```python
from build123d import *

# Parameters (mm, degrees)
ESBO_O1_W                  = 25
ESBO_O1_H                  = 65
ESBO_O1_R                  = 1.75
RESSALTO_EXTRUS_O1_DEPTH   = 5
CORTE_EXTRUS_O3_DEPTH      = 36.178118199
CORTE_EXTRUS_O3_DEPTH_BACK = 36.178118199
FILETE1_R                  = 5
ESBO_O2_R                  = 3.4
CORTE_EXTRUS_O1_DEPTH      = 3
ESBO_O3_W                  = 5.6
ESBO_O3_H                  = 48
CORTE_EXTRUS_O2_DEPTH      = 3


with BuildPart() as part:
    # Esboço1 → Ressalto-extrusão1 (new body)
    with BuildSketch(Plane.XY):
        Rectangle(ESBO_O1_W, ESBO_O1_H)
        with Locations((7.5, 27.5)):
            Circle(ESBO_O1_R, mode=Mode.SUBTRACT)
        with Locations(Location((7.5, -27.5, 0), (0, 0, 180))):
            Circle(ESBO_O1_R, mode=Mode.SUBTRACT)
        with Locations((-7.5, -27.5)):
            Circle(ESBO_O1_R, mode=Mode.SUBTRACT)
        with Locations(Location((-7.5, 27.5, 0), (0, 0, 180))):
            Circle(ESBO_O1_R, mode=Mode.SUBTRACT)
        with BuildLine():
            Line((-1.7, -20), (-1.7, 20))
            ThreePointArc((-1.7, 20), (0, 21.7), (1.7, 20))
            Line((1.7, 20), (1.7, -20))
            ThreePointArc((1.7, -20), (0, -21.7), (-1.7, -20))
        make_face(mode=Mode.SUBTRACT)
    extrude(amount=RESSALTO_EXTRUS_O1_DEPTH)

    # Esboço4 → Corte-extrusão3 (cut, two sides: drawn at the far end of the back side and taken through both)
    with BuildSketch(Plane.XY.offset(5).offset(-CORTE_EXTRUS_O3_DEPTH_BACK)):
        with BuildLine():
            Line((12.5, 27.5), (12.5, -27.5))
            ThreePointArc((12.5, -27.5), (12.365923064, -26.34987273), (11.970882905, -25.261427677))
            ThreePointArc((11.970882905, -25.261427677), (6, 0), (11.970882905, 25.261427677))
            ThreePointArc((11.970882905, 25.261427677), (12.365923064, 26.34987273), (12.5, 27.5))
        make_face()
        with BuildLine():
            Line((-12.5, 27.5), (-12.5, -27.5))
            ThreePointArc((-12.5, -27.5), (-12.365923064, -26.34987273), (-11.970882905, -25.261427677))
            ThreePointArc((-11.970882905, -25.261427677), (-6, 0), (-11.970882905, 25.261427677))
            ThreePointArc((-11.970882905, 25.261427677), (-12.365923064, 26.34987273), (-12.5, 27.5))
        make_face()
    extrude(amount=CORTE_EXTRUS_O3_DEPTH + CORTE_EXTRUS_O3_DEPTH_BACK, mode=Mode.SUBTRACT)

    # Filete1
    filete1_edges = [part.edges().sort_by_distance(p)[0] for p in [
        (-12.5, -32.5, 2.5),
        (12.5, -32.5, 2.5),
        (12.5, 32.5, 2.5),
        (-12.5, 32.5, 2.5),
    ]]
    fillet(filete1_edges, radius=FILETE1_R - 0.0001)  # a hair under: the kernel refuses the full size

    # Esboço2 → Corte-extrusão1 (cut)
    with BuildSketch(Plane.XY.offset(5)):
        with Locations((7.5, 27.5)):
            Circle(ESBO_O2_R)
        with Locations((-7.5, 27.5)):
            Circle(ESBO_O2_R)
        with Locations((-7.5, -27.5)):
            Circle(ESBO_O2_R)
        with Locations((7.5, -27.5)):
            Circle(ESBO_O2_R)
    extrude(amount=-CORTE_EXTRUS_O1_DEPTH, mode=Mode.SUBTRACT)

    # Esboço3 → Corte-extrusão2 (cut)
    with BuildSketch(Plane(origin=(0, 0, 0), x_dir=(-1, 0, 0), z_dir=(0, 0, -1))):
        Rectangle(ESBO_O3_W, ESBO_O3_H)
    extrude(amount=-CORTE_EXTRUS_O2_DEPTH, mode=Mode.SUBTRACT)


solid = part.part
```
The model under review builds one solid part; all positions refer to its coordinate system, in mm. A direction names the side the tool comes from. Give positions to 0.01 mm unless a question says otherwise; leave off trailing zeros. Write each loop counter-clockwise with the first axis right and the second up, starting at its lowest first coordinate (ties: lowest second). Pieces come first, ordered by that corner, then holes. Notation, with made-up numbers: M 79.25,37 L 103.25,37 A20 ccw 103.25,54 Z; hole C 74.5,50.25 d2. An arc over 180 degrees is marked long. Answer in a Markdown table with one row per item.
Item 1: Add section A-A on z = 4.1. State how many separate pieces and enclosed holes the cut face has, plus the area to 3 significant figures.
Check sheet entries:
| item | result |
|---|---|
| separate pieces | 1 |
| enclosed holes | 5 |
| area | 852 mm2 |
Item 2: For P1, Ø2, axis at y = -14, z = 1, coming from the +X side; P2, Ø2, axis at y = 22, z = 1, coming from the -X side; P3, Ø6, axis at x = -7.5, y = -27.5, coming from the +Z side; P4, Ø3, axis at x = 7.5, y = -27.5, coming from the +Z side, all flat-tipped, find the tip position at first contact; note any pin that passes through.
Check sheet entries:
| item | result |
|---|---|
| P1 | x = 8.03 |
| P2 | x = -10.9 |
| P3 | z = 2 |
| P4 | through |
Item 3: Add section B-B on x = -10. Give the boundary of the cut face in (y, z).
Check sheet entries:
| item | result |
|---|---|
| outline | M -31.83,0 L -20.87,0 L -20.87,5 L -25.2,5 L -25.2,2 L -29.8,2 L -29.8,5 L -31.83,5 Z; M 20.87,0 L 31.83,0 L 31.83,5 L 29.8,5 L 29.8,2 L 25.2,2 L 25.2,5 L 20.87,5 Z |
Item 4: Draft analysis for pull direction Y (two halves, no side actions). For faces 1 (the face through (0, 32.5, 2)), 2 (the face through (12.36, 26.33, 2.47)), 3 (the face through (-11.07, -31, 2.54)), state which applies: +Y half, -Y half, draft (parallel to the pull), parting line (faces both ways), or undercut.
Check sheet entries:
| item | result |
|---|---|
| face 1 | +Y half |
| face 2 | undercut |
| face 3 | -Y half |
Item 5: Tool access review of faces 4 (the face through (12.37, -26.37, 2.47)), 5 (the face through (-12.36, 26.33, 2.47)), 6 (the face through (-1.7, 0, 4)), 7 (the face through (11, -31.07, 2.54)), 8 (the face through (10.743, -26.479, 3.521)): name each direction out of +Z, -Z, +X, -X, +Y, -Y from which nothing blocks a thin tool from reaching the whole face with its end or side.
Check sheet entries:
| item | result |
|---|---|
| face 4 | +Z, -Z, +X |
| face 5 | +Z, -Z, -X |
| face 6 | +Z, -Z |
| face 7 | +Z, -Z, +X, -Y |
| face 8 | +Z |
Item 6: For line 1 along X through (y, z) = (27.5, 1.65); line 2 along Y through (x, z) = (5.5, 4.1); line 3 along Y through (x, z) = (0.5, 0.85), list the stretches that pass through material, from the lowest coordinate up.
Check sheet entries:
| item | result |
|---|---|
| line 1 | -12.5 to -9.25, -5.75 to 5.75, 9.25 to 12.5 |
| line 2 | -32.5 to -30.25, -24.75 to 24.75, 30.25 to 32.5 |
| line 3 | -32.5 to -24, 24 to 32.5 |
Item 7: Add section C-C on y = -7. Give the boundary of the cut face in (x, z), plus the area to 3 significant figures.
Check sheet entries:
| item | result |
|---|---|
| outline | M -6.44,0 L -2.8,0 L -2.8,3 L -1.7,3 L -1.7,5 L -6.44,5 Z; M 1.7,3 L 2.8,3 L 2.8,0 L 6.44,0 L 6.44,5 L 1.7,5 Z |
| area | 40.8 mm2 |
